CAD build for the part. Positions are in the model's coordinates, mm. A direction names the side the tool comes from. Coordinates: 2 decimals unless noted, no trailing zeros. Order: outer loops, then holes, each group sorted by start corner. A loop starts at its lowest first (then second) coordinate and runs counter-clockwise, first axis right, second up. Notation, with made-up numbers: M 42,73 L 82,73 A31 cw 82,97 Z; hole C 34,80.25 d11. An arc over 180 degrees is marked long. One line per item, written item: value.
from build123d import *

# Parameters (mm, degrees)
F0_W      = 0.6
F0_H      = 17.1
F2_R      = 0.4
F3_R      = 1
F4_R      = 6.45
F5_DEPTH  = 4.5
F6_R      = 0.5
F7_R      = 4.8
F8_DEPTH  = 0.6
F4_R_2    = 1.25
F9_DEPTH  = 25
F10_R     = 17.1
F11_DEPTH = 0.6


with BuildPart() as f1:
    # F0 (on Top) → F1 (revolve)
    with BuildSketch(Plane.XY):
        with Locations((0.3, 8.55)):
            Rectangle(F0_W, F0_H)
        Polygon((0, 17.7), (0, 17.1), (0.6, 17.1), (57, 17.1), (57, 17.7), align=None)
    revolve(axis=Axis((0.3, 0, 0), (1, 0, 0)))

    # F2
    f2_edges = [f1.edges().sort_by_distance(p)[0] for p in [
        (0.6, -17.1, 0),
    ]]
    fillet(f2_edges, radius=F2_R)

    # F3
    f3_edges = [f1.edges().sort_by_distance(p)[0] for p in [
        (0, -17.7, 0),
    ]]
    fillet(f3_edges, radius=F3_R)

    # F4 (on Right) → F5 (join)
    with BuildSketch(Plane.YZ):
        Circle(F4_R)
    extrude(amount=-F5_DEPTH)

    # F6
    f6_edges = [f1.edges().sort_by_distance(p)[0] for p in [
        (0, -6.45, 0),
        (-4.5, -6.45, 0),
    ]]
    fillet(f6_edges, radius=F6_R)

    # F7 (on face) → F8 (cut)
    with BuildSketch(Plane(origin=(-4.5, 0, 0), x_dir=(0, -1, 0), z_dir=(-1, 0, 0))):
        Circle(F7_R)
    extrude(amount=-F8_DEPTH, mode=Mode.SUBTRACT)

    # F4 (on Right) → F9 (cut)
    with BuildSketch(Plane.YZ):
        with Locations((0, -12.5)):
            Circle(F4_R_2)
        with Locations((0, 12.5)):
            Circle(F4_R_2)
    extrude(amount=F9_DEPTH, mode=Mode.SUBTRACT)

    # F10 (on face) → F11 (join)
    with BuildSketch(Plane.YZ.offset(57)):
        Circle(F10_R)
    extrude(amount=-F11_DEPTH)


solid = f1.part
Q1. Mould opens along Z. For faces 4 (the face through (0, -0.2, -7.2)), 5 (the face through (0.3, -0.16, 13.74)), 6 (the face through (28.61, 16.88, 5.32)) say: released by +Z, released by -Z, zero draft, split by the parting line, or undercut.
Recorded:
face 4: zero draft
face 5: undercut
face 6: split by the parting line
Q2. Drill centre lines: line 1 along Z through (x, y) = (41.5, 0.5); line 2 along X through (y, z) = (4, 7); line 3 along Z through (x, y) = (0.2, 0). Where is each one in solid material? Low to high.
Recorded:
line 1: z = -17.69 to -17.09, 17.09 to 17.69
line 2: x = 0 to 0.6, 56.4 to 57
line 3: z = -17.3 to -13.75, -11.25 to 11.25, 13.75 to 17.3
Q3. Which spindle directions (+Z, -Z, +X, -X, +Y, -Y) get a long thin tool onto all of the face, cutting with end or side? Do faces 1 (the face through (57, 0, 0)), 2 (the face through (0.6, 0, 0)), 3 (the face through (-2.226, -1.398, -6.297)). Say none if no direction does.
Recorded:
face 1: +Z, -Z, +X, +Y, -Y
face 2: none
face 3: -X
Q4. Slice it at C-C (x = 7). List the corners of the cut face in (y, z).
Recorded:
outline: C 0,0 d35.4; hole C 0,0 d34.2
Q5. Pin check, flat tips, straight feed: pin 1 Ø7.5 at (y, z) = (2.5, 2) entering from -X; pin 2 Ø10 at (x, z) = (4.5, -11) entering from -Y; pin 3 Ø2 at (x, y) = (42, -13) entering from -Z; pin 4 Ø4 at (x, z) = (29, -6.5) entering from -Y. Stop position of each tip, or through.
Recorded:
pin 1: stops at x = -4.5
pin 2: stops at y = -16.65
pin 3: stops at z = -13.01
pin 4: stops at y = -17.12
Q6. Slice it at B-B (z = 0). List the corners of the cut face in (x, y), plus the area to 3 significant figures.
Recorded:
outline: M -4.5,-5.95 A0.5 ccw -4,-6.45 L -0.5,-6.45 A0.5 cw 0,-6.95 L 0,-16.7 A1 ccw 1,-17.7 L 57,-17.7 L 57,17.7 L 1,17.7 A1 ccw 0,16.7 L 0,6.95 A0.5 cw -0.5,6.45 L -4,6.45 A0.5 ccw -4.5,5.95 L -4.5,4.8 L -3.9,4.8 L -3.9,-4.8 L -4.5,-4.8 Z; hole M 0.6,-16.7 A0.4 ccw 1,-17.1 L 56.4,-17.1 L 56.4,17.1 L 1,17.1 A0.4 ccw 0.6,16.7 Z
area: 161 mm^2
